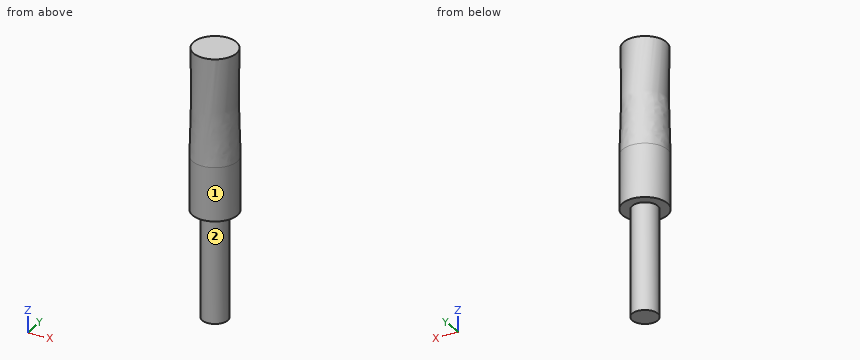
from build123d import *

# Parameters (mm, degrees)
ESBO_O1_R                = 4.2
RESSALTO_EXTRUS_O1_DEPTH = 10
ESBO_O3_R                = 2.4
RESSALTO_EXTRUS_O2_DEPTH = 20


with BuildPart() as part:
    # Esboço1 → Ressalto-extrusão1 (new body)
    with BuildSketch(Plane.XY):
        Circle(ESBO_O1_R)
    extrude(amount=RESSALTO_EXTRUS_O1_DEPTH)

    # Loft1: read off the stored shape, not the designer's step
    # Loft1: loft between two sections, ruled curve by curve
    loft1_from = [
        Edge.make_bspline([(1.94680537, -3.494273723, 30), (-5.041742075, -7.387884464, 30), (-8.935352816, -0.399337018, 30), (-1.94680537, 3.494273723, 30), (5.041742075, 7.387884464, 30), (8.935352816, 0.399337018, 30), (1.94680537, -3.494273723, 30)], [0, 0, 0, 0, 0.5, 0.5, 0.5, 1, 1, 1, 1], 3, [1, 0.333333333, 0.333333333, 1, 0.333333333, 0.333333333, 1]),
    ]
    loft1_to = [
        Edge.make_bspline([(-0.110822525, -4.198537646, 10), (-8.507897818, -3.976892596, 10), (-8.286252768, 4.420182696, 10), (0.110822525, 4.198537646, 10), (8.507897818, 3.976892596, 10), (8.286252768, -4.420182696, 10), (-0.110822525, -4.198537646, 10)], [0, 0, 0, 0, 0.5, 0.5, 0.5, 1, 1, 1, 1], 3, [1, 0.333333333, 0.333333333, 1, 0.333333333, 0.333333333, 1]),
    ]
    loft1 = Solid(Shell([*[Face.make_surface_from_curves(loft1_from[k], loft1_to[k]) for k in range(1)], Face(Wire(loft1_from)), Face(Wire(loft1_to))]))
    add(loft1)

    # Esboço3 → Ressalto-extrusão2 (add)
    with BuildSketch(Plane(origin=(0, 0, 0), x_dir=(-1, 0, 0), z_dir=(0, 0, -1))):
        Circle(ESBO_O3_R)
    extrude(amount=RESSALTO_EXTRUS_O2_DEPTH)


solid = part.part
CAD build for the part. Positions are in the model's coordinates, mm. Face numbers are marked on the shaded views. A direction names the side the tool comes from. Round coordinates to 2 decimals unless told otherwise and drop trailing zeros. Order: outer loops, then holes, each group sorted by start corner. A loop starts at its lowest first (then second) coordinate and runs counter-clockwise, first axis right, second up. Notation, with made-up numbers: (44, 13.5) -> (86, 13.5) arc R36 ccw to (86, 49.5) -> close; hole circle Ø5 at (48.5, 58.5). An arc over 180 degrees is marked (long way). Write item = value, one per line. Start each with the question number.
(1) Cut at A-A, the plane z = -10.5. List the corners of the cut face in (x, y), then the cut area to 3 significant figures.
(2) Cut at B-B, the plane z = 3. List the corners of the cut face in (x, y).
(3) Which spindle directions (+Z, -Z, +X, -X, +Y, -Y) get a long thin tool onto all of the face, cutting with end or side? Do the marked faces 1 and 2. Say none if no direction does.
(4) Pin check, flat tips, straight feed: P1, Ø3, axis at x = -1, z = -3.5, coming from the -Y side; P2, Ø1, axis at y = -2.5, z = 15, coming from the +X side; P3, Ø1, axis at x = -3, y = -2, coming from the -Z side; P4, Ø5, axis at x = -1, y = -2.5, coming from the -Z side. Stop position of each tip, or through.
(5) Probe line 1 (Z direction, x = 3, y = -1); line 2 (X direction, y = 1.25, z = 10); line 3 (Y direction, x = 2.5, z = 18.5). List the from-to ranges inside material, lowest first. Write a range as [from, to].
Model answer:
q1.outline = circle Ø4.8 at (0, 0)
q1.area = 18.1 mm2
q2.outline = circle Ø8.4 at (0, 0)
q3.face_1 = +Z, -Z
q3.face_2 = -Z
q4.P1 = -2.4
q4.P2 = 3.51
q4.P3 = 0
q4.P4 = -20
q5.line_1 = [0, 30]
q5.line_2 = [-4.01, 4.01]
q5.line_3 = [-3.09, 3.09]
